Geometry check sheet. Reference: the model listing, model coordinates, mm. A direction names the side the tool comes from. Give positions to 0.01 mm unless a question says otherwise; leave off trailing zeros. Order: outer loops, then holes, each group sorted by start corner. A loop starts at its lowest first (then second) coordinate and runs counter-clockwise, first axis right, second up.
from build123d import *

# Parameters (mm, degrees)
F0_W     = 406.4
F0_H     = 457.2
F1_DEPTH = 101.6
F2_W     = 82.55
F2_H     = 76.2
F3_DEPTH = 406.4
F4_W     = 368.3
F4_H     = 63.5
F5_DEPTH = 361.95
F6_W     = 215.9
F6_H     = 311.15
F7_DEPTH = 101.6


with BuildPart() as f1:
    # F0 (on Front) → F1 (new body)
    with BuildSketch(Plane.XZ):
        with Locations((3.443759, -38.172014)):
            Rectangle(F0_W, F0_H)
    extrude(amount=F1_DEPTH)

    # F2 (on face) → F3 (cut)
    with BuildSketch(Plane.YZ.offset(206.643759)):
        with Locations((-60.325, 152.327986)):
            Rectangle(F2_W, F2_H)
    extrude(amount=-F3_DEPTH, mode=Mode.SUBTRACT)

    # F4 (on face) → F5 (cut)
    with BuildSketch(Plane.XY.offset(114.227986)):
        with Locations((3.443759, -50.8)):
            Rectangle(F4_W, F4_H)
    extrude(amount=-F5_DEPTH, mode=Mode.SUBTRACT)

    # F6 (on face) → F7 (cut)
    with BuildSketch(Plane(origin=(0, 0, 0), x_dir=(-1, 0, 0), z_dir=(0, 1, 0))):
        with Locations((-3.443759, 34.852986)):
            Rectangle(F6_W, F6_H)
    extrude(amount=-F7_DEPTH, mode=Mode.SUBTRACT)


solid = f1.part
Item 1: Sectioned sample at A-A (z = -29.5). Enter the section's corners in (x, y).
Reported:
outline: (-199.76, -101.6) - (-104.51, -101.6) - (-104.51, -82.55) - (-180.71, -82.55) - (-180.71, -19.05) - (-104.51, -19.05) - (-104.51, 0) - (-199.76, 0) - close; (111.39, -101.6) - (206.64, -101.6) - (206.64, 0) - (111.39, 0) - (111.39, -19.05) - (187.59, -19.05) - (187.59, -82.55) - (111.39, -82.55) - close
Item 2: Sectioned sample at C-C (x = -149). Enter the section's corners in (y, z).
Reported:
outline: (-101.6, -266.77) - (0, -266.77) - (0, 190.43) - (-19.05, 190.43) - (-19.05, -247.72) - (-82.55, -247.72) - (-82.55, 114.23) - (-101.6, 114.23) - close
Item 3: Set-up check for faces 4 (the flat face through (-173, -88, 114.228)), 5 (the flat face through (5, -9, -120.722)), 6 (the flat face through (206.644, -50, -41)), 7 (the flat face through (187.594, -51, -64)): record each of +Z, -Z, +X, -X, +Y, -Y from which the full face is reachable in a straight line by a thin tool's end or side.
Reported:
face 4: +Z, +X, -X, -Y
face 5: +Z, +Y, -Y
face 6: +Z, -Z, +X, +Y, -Y
face 7: +Z
Item 4: Sectioned sample at B-B (y = -89). Enter the section's corners in (x, z), and give its area (3 significant figures).
Reported:
outline: (-199.76, -266.77) - (206.64, -266.77) - (206.64, 114.23) - (111.39, 114.23) - (111.39, -120.72) - (-104.51, -120.72) - (-104.51, 114.23) - (-199.76, 114.23) - close
area: 104,000 mm2
Item 5: Draft check along Y on faces 1 (the flat face through (-199.756, -50, -41)), 2 (the flat face through (1, -82.55, -145)), 3 (the flat face through (1, -101.6, -158)). Enter one of: released by +Y, released by -Y, zero draft, split by the parting line, or undercut.
Reported:
face 1: zero draft
face 2: undercut
face 3: released by -Y
Item 6: Sectioned sample at D-D (z = -199). Enter the section's corners in (x, y), and give its area (3 significant figures).
Reported:
outline: (-199.76, -101.6) - (206.64, -101.6) - (206.64, 0) - (-199.76, 0) - close; hole (-180.71, -82.55) - (187.59, -82.55) - (187.59, -19.05) - (-180.71, -19.05) - close
area: 17,900 mm2
Item 7: Scan lines: L1, parallel to X at y = -70, z = 88; L2, parallel to Y at x = -148, z = 101.5; L3, parallel to X at y = -4.5, z = -71. Record each from-to range of solid material in increasing order.
Reported:
L1: x = -199.76 to -180.71, 187.59 to 206.64
L2: y = -101.6 to -82.55, -19.05 to 0
L3: x = -199.76 to -104.51, 111.39 to 206.64
Item 8: Gauge pin test, flat ends, axial feed: pin 1 (5.5 mm diameter, centred on x = 55, y = -93.5, fed in from +Z); pin 2 (2 mm diameter, centred on x = 49, y = -48.5, fed in from +Z). Record the tip position at first contact, or that the pin passes through.
Reported:
pin 1: stops at z = -120.72
pin 2: stops at z = -247.72
